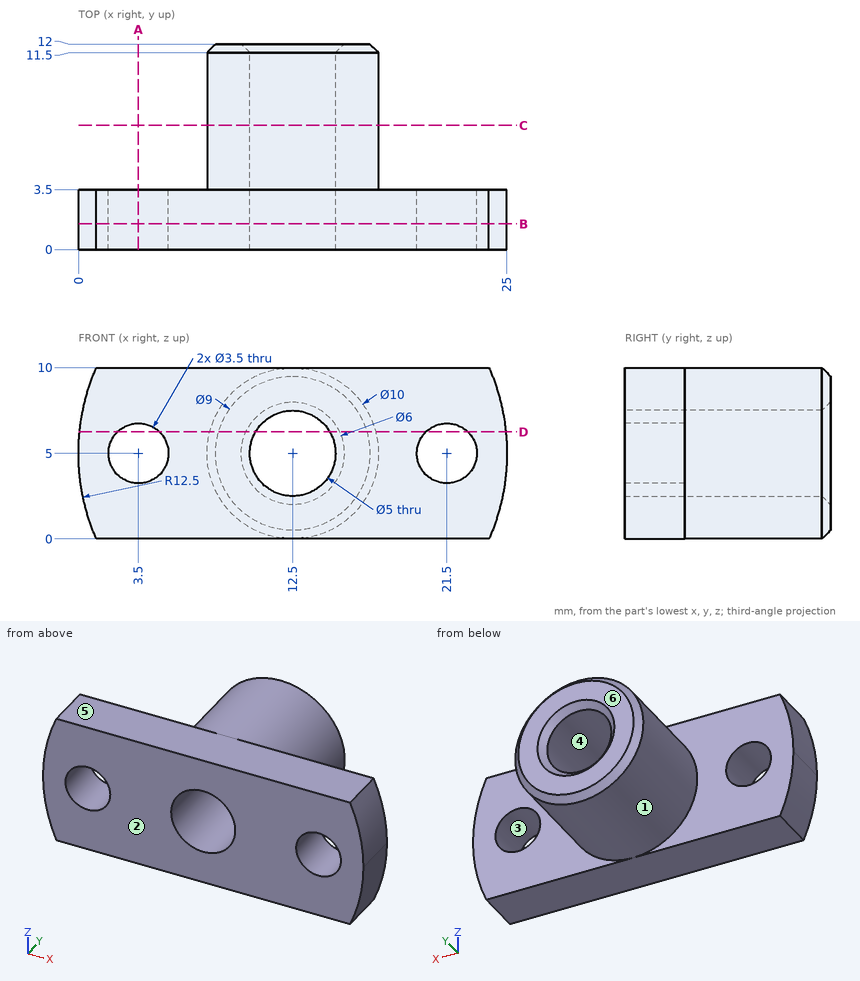
Part print with two shaded views. Sizes in mm from the minimum x, y, z corner. A direction names the side the tool comes from. Coordinates: 2 decimals unless noted, no trailing zeros. Order: outer loops, then holes, each group sorted by start corner. A loop starts at its lowest first (then second) coordinate and runs counter-clockwise, first axis right, second up.
(1) Mould opens along Z. For the marked faces 3, 4, 5 and 6 say: released by +Z, released by -Z, zero draft, split by the parting line, or undercut.
Solution:
face 3: undercut
face 4: undercut
face 5: released by +Z
face 6: zero draft
(2) Which spindle directions (+Z, -Z, +X, -X, +Y, -Y) get a long thin tool onto all of the face, cutting with end or side? Do the marked faces 1 and 2. Say none if no direction does.
Solution:
face 1: +Y
face 2: +Z, -Z, +X, -X, -Y
(3) Drill centre lines: L1, parallel to X at y = 6.25, z = 5; L2, parallel to Y at x = 21, z = 6.75; L3, parallel to X at y = 9.5, z = 9. Where is each one in solid material? Low to high.
Solution:
L1: x = 7.5 to 10, 15 to 17.5
L2: y = 0 to 3.5
L3: x = 9.5 to 15.5
(4) Saw through at D-D, the plane z = 6.25. Count the separate pieces of the cut face and the enclosed holes in it, and give its area (3 significant figures).
Solution:
separate pieces: 4
enclosed holes: 0
area: 99.7 mm2
(5) Saw through at B-B, the plane y = 1.5. Write the cut outline in (x, z).
Solution:
outline: (1.04, 0) - (23.96, 0) arc R12.5 ccw to (23.96, 10) - (1.04, 10) arc R12.5 ccw to start; hole circle Ø3.5 at (3.5, 5); hole circle Ø5 at (12.5, 5); hole circle Ø3.5 at (21.5, 5)
(6) Saw through at C-C, the plane y = 7.25. Write the cut outline in (x, z), and give its area (3 significant figures).
Solution:
outline: circle Ø10 at (12.5, 5); hole circle Ø5 at (12.5, 5)
area: 58.9 mm2
(7) Pin check, flat tips, straight feed: pin 1 Ø3 at (x, z) = (3.5, 5) entering from +Y; pin 2 Ø1 at (x, z) = (21.5, 9) entering from +Y; pin 3 Ø5 at (y, z) = (8, 2.5) entering from -X. Stop position of each tip, or through.
Solution:
pin 1: passes through
pin 2: stops at y = 3.5
pin 3: stops at x = 7.5
(8) Saw through at A-A, the plane x = 3.5. Write the cut outline in (y, z).
Solution:
outline: (0, 0) - (3.5, 0) - (3.5, 3.25) - (0, 3.25) - close; (0, 6.75) - (3.5, 6.75) - (3.5, 10) - (0, 10) - close
